Read the model definition and answer for the solid it produces. Units are mm, in the model's axes. A direction names the side the tool comes from. Give positions to 0.01 mm unless a question says otherwise; leave off trailing zeros. Write each loop counter-clockwise with the first axis right and the second up, starting at its lowest first coordinate (ties: lowest second). Pieces come first, ordered by that corner, then holes. Notation, with made-up numbers: M 52.5,62 L 92.5,62 A29 cw 92.5,89 Z; hole C 52,79 d11. An arc over 180 degrees is marked long. Write each question's results on one line, items separated by ' | '. Start each with the question number.
```python
from build123d import *

# Parameters (mm, degrees)
BOSS_EXTRUDE1_DEPTH     = 10
SKETCH3_R               = 10
BOSS_EXTRUDE2_DEPTH     = 60
SKETCH4_R               = 7.5
CUT_EXTRUDE1_DEPTH      = 32
CUT_EXTRUDE1_DEPTH_BACK = 12


with BuildPart() as part:
    # Sketch2 → Boss-Extrude1 (new body, symmetric)
    with BuildSketch(Plane.XY):
        Polygon((0, 25), (0, -25), (40, -25), (40, -10), (15, -10), (15, 10), (40, 10), (40, 25), align=None)
    extrude(amount=BOSS_EXTRUDE1_DEPTH, both=True)

    # Sketch3 → Boss-Extrude2 (add)
    with BuildSketch(Plane.ZY):
        Circle(SKETCH3_R)
    extrude(amount=BOSS_EXTRUDE2_DEPTH)

    # Sketch4 → Cut-Extrude1 (cut, two sides)
    with BuildSketch(Plane.XZ.offset(-10)) as cut_extrude1_sk:
        with Locations((30, 0)):
            Circle(SKETCH4_R)
    extrude(amount=CUT_EXTRUDE1_DEPTH, mode=Mode.SUBTRACT)
    extrude(cut_extrude1_sk.sketch, amount=-CUT_EXTRUDE1_DEPTH_BACK, mode=Mode.SUBTRACT)


solid = part.part
```
Item 1: Section A-A, the plane x = 30 is taken. Determine the outline of the cut face in (y, z), then the cut area to 3 significant figures.
Item 2: Section C-C, the plane x = 18 is taken. Determine the outline of the cut face in (y, z).
Item 3: Determine the mould class of faces 1 (the flat face through (15, 0, 0)), 2 (the flat face through (30, 22, 0)), 3 (the flat face through (11, 0, -10)) for opening direction X: +X half, -X half, draft (parallel to the pull), parting line (faces both ways), or undercut.
Item 4: Given P1, Ø10, axis at y = 18.5, z = -1, coming from the -X side; P2, Ø8, axis at x = -7.5, z = 2, coming from the +Y side; P3, Ø4, axis at x = -33, y = 6.5, coming from the -Z side, each flat-ended and moving along its own axis, determine where each tip first touches the part or whether it passes through.
Item 5: Section B-B, the plane y = 15.5 is taken. Determine the outline of the cut face in (x, z), then the cut area to 3 significant figures.
Item 6: Straight lines are drawn through the part: line 1 (Y direction, x = 30, z = 4); line 2 (Z direction, x = 30, y = -13); line 3 (X direction, y = -15.5, z = 0). For each, find the intervals that lie inside material, in ascending order.
Item 7: Section D-D, the plane z = 0 is taken. Determine the outline of the cut face in (x, y), then the cut area to 3 significant figures.
Item 8: For faces 4 (the cylindrical face through (-29.58, -9.76, -2.17)), 5 (the flat face through (30, -22, 0)), 6 (the flat face through (22, -10, 0)), determine the directions among +Z, -Z, +X, -X, +Y, -Y from which every point of the face is accessible in a straight line to the end or side of a thin tool.
Worked out:
1) outline: M -25,-10 L -10,-10 L -10,-7.5 L -22,-7.5 L -22,7.5 L -10,7.5 L -10,10 L -25,10 Z; M 10,-10 L 25,-10 L 25,10 L 10,10 L 10,7.5 L 22,7.5 L 22,-7.5 L 10,-7.5 Z | area: 240 mm²
2) outline: M -25,-10 L -10,-10 L -10,10 L -25,10 Z; M 10,-10 L 25,-10 L 25,10 L 10,10 Z
3) face 1: +X half | face 2: undercut | face 3: draft
4) P1: stops at x = 0 | P2: stops at y = 10 | P3: stops at z = -8.93
5) outline: M 0,-10 L 40,-10 L 40,10 L 0,10 Z; hole C 30,0 d15 | area: 623 mm²
6) line 1: y = -25 to -22, 22 to 25 | line 2: z = -10 to -7.5, 7.5 to 10 | line 3: x = 0 to 22.5, 37.5 to 40
7) outline: M -60,-10 L 0,-10 L 0,-25 L 40,-25 L 40,-10 L 37.5,-10 L 37.5,-22 L 22.5,-22 L 22.5,-10 L 15,-10 L 15,10 L 22.5,10 L 22.5,22 L 37.5,22 L 37.5,10 L 40,10 L 40,25 L 0,25 L 0,10 L -60,10 Z | area: 2,340 mm²
8) face 4: -X | face 5: none | face 6: +Z, -Z, +X
